```python
from build123d import *

# Parameters (mm, degrees)
SKETCH2_R           = 10.25
BOSS_EXTRUDE1_DEPTH = 1
SKETCH3_W           = 8
SKETCH3_H           = 8.5
BOSS_EXTRUDE2_DEPTH = 8
CUT_EXTRUDE1_START  = 4
SKETCH4_R           = 1.5
CUT_EXTRUDE1_DEPTH  = 2
SKETCH4_3_R         = 1.5
CUT_EXTRUDE3_DEPTH  = 8


with BuildPart() as part:
    # Sketch1 → Revolve1 (revolve)
    with BuildSketch(Plane.XY):
        Polygon((-6.674207745, -1.25), (-6.674207745, 0), (-10.25, 0), (-10.25, -36.5), (-9, -36.5), (-9, -1.25), align=None)
    revolve(axis=Axis((0, 9.278019649, 0), (0, -1, 0)))

    # Sketch2 → Boss-Extrude1 (add)
    with BuildSketch(Plane.XZ.offset(36.5)):
        Circle(SKETCH2_R)
    extrude(amount=BOSS_EXTRUDE1_DEPTH)

    # Sketch3 → Boss-Extrude2 (add)
    with BuildSketch(Plane.XZ.offset(37.5)):
        Rectangle(SKETCH3_W, SKETCH3_H)
    extrude(amount=BOSS_EXTRUDE2_DEPTH)

    # Sketch4 → Cut-Extrude1 (cut, symmetric)
    with BuildSketch(Plane(origin=(4, 0, -0.2768318), x_dir=(0, 0, 1), z_dir=(-1, 0, 0)).offset(CUT_EXTRUDE1_START)):
        with BuildLine():
            Line((4.5268318, -44.6), (4.5268318, -38.4))
            Line((4.5268318, -38.4), (-0.4731682, -38.4))
            ThreePointArc((-0.4731682, -38.4), (-3.5731682, -41.5), (-0.4731682, -44.6))
            Line((-0.4731682, -44.6), (4.5268318, -44.6))
        make_face()
        with Locations((2.3268318, -41.5)):
            Circle(SKETCH4_R, mode=Mode.SUBTRACT)
    extrude(amount=CUT_EXTRUDE1_DEPTH, both=True, mode=Mode.SUBTRACT)

    # Sketch4<3> → Cut-Extrude3 (cut)
    with BuildSketch(Plane(origin=(4, 0, -0.2768318), x_dir=(0, 0, 1), z_dir=(-1, 0, 0))):
        with Locations((2.3268318, -41.5)):
            Circle(SKETCH4_3_R)
    extrude(amount=CUT_EXTRUDE3_DEPTH, mode=Mode.SUBTRACT)


solid = part.part
```
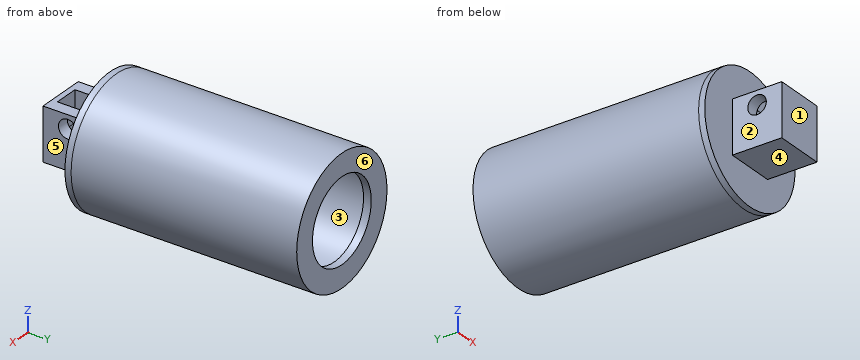
Can you work these out from the model? Positions are in its coordinate system, mm. Face numbers are marked on the shaded views. A direction names the side the tool comes from. Round coordinates to 2 decimals unless told otherwise and drop trailing zeros. Order: outer loops, then holes, each group sorted by start corner. A loop starts at its lowest first (then second) coordinate and runs counter-clockwise, first axis right, second up.
(1) If we section it at B-B (z = 2.5): Please give me the cut outline in (x, y).
Results are:
outline: (-9.94, -37.5) - (-4, -37.5) - (-4, -40.07) - (-2, -40.07) - (-2, -38.4) - (2, -38.4) - (2, -40.07) - (4, -40.07) - (4, -37.5) - (9.94, -37.5) - (9.94, 0) - (6.19, 0) - (6.19, -1.25) - (8.65, -1.25) - (8.65, -36.5) - (-8.65, -36.5) - (-8.65, -1.25) - (-6.19, -1.25) - (-6.19, 0) - (-9.94, 0) - close; (-4, -45.5) - (4, -45.5) - (4, -42.93) - (2, -42.93) - (2, -44.6) - (-2, -44.6) - (-2, -42.93) - (-4, -42.93) - close
(2) If we section it at D-D (x = -4.5): Please give me the cut outline in (y, z).
Results are:
outline: (-37.5, -9.21) - (0, -9.21) - (0, -4.93) - (-1.25, -4.93) - (-1.25, -7.79) - (-36.5, -7.79) - (-36.5, 7.79) - (-1.25, 7.79) - (-1.25, 4.93) - (0, 4.93) - (0, 9.21) - (-37.5, 9.21) - close
(3) I'm going to push flat-ended pins straight in: pin 1 (8 mm diameter, centred on x = 1.5, z = 0.5, fed in from +Y); pin 2 (2.5 mm diameter, centred on y = -39.5, z = -2, fed in from -X); pin 3 (5 mm diameter, centred on y = -6, z = 5, fed in from +X). Where does each tip first touch, or does it pass through?
Results are:
pin 1: stops at y = -36.5
pin 2: stops at x = -4
pin 3: stops at x = 9.94
(4) If we section it at C-C (x = 8.5): Please give me the cut outline in (y, z), plus the area to 3 significant figures.
Results are:
outline: (-37.5, -5.73) - (0, -5.73) - (0, 5.73) - (-37.5, 5.73) - close; hole (-36.5, -2.96) - (-1.25, -2.96) - (-1.25, 2.96) - (-36.5, 2.96) - close
area: 221 mm2
(5) We'd pull the mould along Y, two halves only. Please class the marked faces 1, 2 and 3: +Y half, -Y half, draft (parallel to the pull), parting line (faces both ways), or undercut.
Results are:
face 1: -Y half
face 2: draft
face 3: undercut
(6) If we section it at A-A (y = -41.5): Please give me the cut outline in (x, z), plus the area to 3 significant figures.
Results are:
outline: (-4, -4.25) - (4, -4.25) - (4, 0.55) - (2, 0.55) - (2, -3.85) - (-2, -3.85) - (-2, 0.55) - (-4, 0.55) - close; (-4, 3.55) - (-2, 3.55) - (-2, 4.25) - (-4, 4.25) - close; (2, 3.55) - (4, 3.55) - (4, 4.25) - (2, 4.25) - close
area: 23.6 mm2
(7) If I drill on L1, parallel to Y at x = 8.5, z = -2.25; L2, parallel to Z at x = 0, y = -0.8; L3, parallel to Z at x = -0.25, y = -26, over which ranges is the centre line in solid material (lowest first)?
Results are:
L1: y = -37.5 to -36.5, -1.25 to 0
L2: z = -10.25 to -6.67, 6.67 to 10.25
L3: z = -10.25 to -9, 9 to 10.25
(8) On a 3-axis mill with a long thin cutter (end or side, diameter ignored), from which of +Z, -Z, +X, -X, +Y, -Y can I reach the whole of each face in a straight line? I mean the marked faces 4, 5 and 6. Say none if no direction works.
Results are:
face 4: -Z, +X, -X, -Y
face 5: +Z, -Z, +X, -Y
face 6: +Z, -Z, +X, -X, +Y
